from build123d import *

# Parameters (mm, degrees)
BOSS_EXTRUDE1_DEPTH = 3


with BuildPart() as part:
    # Base_Sketch → Boss-Extrude1 (new body)
    with BuildSketch(Plane.XY):
        with BuildLine():
            Line((-8.603981625, 52.439957176), (-8.603981625, 50.01533765))
            ThreePointArc((-8.603981625, 50.01533765), (-15.682612465, 48.266118202), (-22.437510505, 45.520551648))
            Line((-22.437510505, 45.520551648), (-23.862666105, 47.48211005))
            Line((-23.862666105, 47.48211005), (-24.825537526, 47.634613901))
            Line((-24.825537526, 47.634613901), (-37.631696962, 38.33039445))
            Line((-37.631696962, 38.33039445), (-37.784200813, 37.36752303))
            Line((-37.784200813, 37.36752303), (-36.359045213, 35.405964628))
            ThreePointArc((-36.359045213, 35.405964628), (-41.057612465, 29.830101554), (-44.908636245, 23.638462104))
            Line((-44.908636245, 23.638462104), (-47.214586445, 24.387710742))
            Line((-47.214586445, 24.387710742), (-48.083205302, 23.945127328))
            Line((-48.083205302, 23.945127328), (-52.974722942, 8.890584019))
            Line((-52.974722942, 8.890584019), (-52.532139528, 8.021965161))
            Line((-52.532139528, 8.021965161), (-50.226189328, 7.272716523))
            ThreePointArc((-50.226189328, 7.272716523), (-50.75, 0), (-50.226189328, -7.272716523))
            Line((-50.226189328, -7.272716523), (-52.532139528, -8.021965161))
            Line((-52.532139528, -8.021965161), (-52.974722942, -8.890584019))
            Line((-52.974722942, -8.890584019), (-48.083205302, -23.945127328))
            Line((-48.083205302, -23.945127328), (-47.214586445, -24.387710742))
            Line((-47.214586445, -24.387710742), (-44.908636245, -23.638462104))
            ThreePointArc((-44.908636245, -23.638462104), (-41.057612465, -29.830101554), (-36.359045213, -35.405964628))
            Line((-36.359045213, -35.405964628), (-37.784200813, -37.36752303))
            Line((-37.784200813, -37.36752303), (-37.631696962, -38.33039445))
            Line((-37.631696962, -38.33039445), (-24.825537526, -47.634613901))
            Line((-24.825537526, -47.634613901), (-23.862666105, -47.48211005))
            Line((-23.862666105, -47.48211005), (-22.437510505, -45.520551648))
            ThreePointArc((-22.437510505, -45.520551648), (-15.682612465, -48.266118202), (-8.603981625, -50.01533765))
            Line((-8.603981625, -50.01533765), (-8.603981625, -52.439957176))
            Line((-8.603981625, -52.439957176), (-7.914641797, -53.129297004))
            Line((-7.914641797, -53.129297004), (7.914641797, -53.129297004))
            Line((7.914641797, -53.129297004), (8.603981625, -52.439957176))
            Line((8.603981625, -52.439957176), (8.603981625, -50.01533765))
            ThreePointArc((8.603981625, -50.01533765), (15.682612465, -48.266118202), (22.437510505, -45.520551648))
            Line((22.437510505, -45.520551648), (23.862666105, -47.48211005))
            Line((23.862666105, -47.48211005), (24.825537526, -47.634613901))
            Line((24.825537526, -47.634613901), (37.631696962, -38.33039445))
            Line((37.631696962, -38.33039445), (37.784200813, -37.36752303))
            Line((37.784200813, -37.36752303), (36.359045213, -35.405964628))
            ThreePointArc((36.359045213, -35.405964628), (41.057612465, -29.830101554), (44.908636245, -23.638462104))
            Line((44.908636245, -23.638462104), (47.214586445, -24.387710742))
            Line((47.214586445, -24.387710742), (48.083205302, -23.945127328))
            Line((48.083205302, -23.945127328), (52.974722942, -8.890584019))
            Line((52.974722942, -8.890584019), (52.532139528, -8.021965161))
            Line((52.532139528, -8.021965161), (50.226189328, -7.272716523))
            ThreePointArc((50.226189328, -7.272716523), (50.75, 0), (50.226189328, 7.272716523))
            Line((50.226189328, 7.272716523), (52.532139528, 8.021965161))
            Line((52.532139528, 8.021965161), (52.974722942, 8.890584019))
            Line((52.974722942, 8.890584019), (48.083205302, 23.945127328))
            Line((48.083205302, 23.945127328), (47.214586445, 24.387710742))
            Line((47.214586445, 24.387710742), (44.908636245, 23.638462104))
            ThreePointArc((44.908636245, 23.638462104), (41.057612465, 29.830101554), (36.359045213, 35.405964628))
            Line((36.359045213, 35.405964628), (37.784200813, 37.36752303))
            Line((37.784200813, 37.36752303), (37.631696962, 38.33039445))
            Line((37.631696962, 38.33039445), (24.825537526, 47.634613901))
            Line((24.825537526, 47.634613901), (23.862666105, 47.48211005))
            Line((23.862666105, 47.48211005), (22.437510505, 45.520551648))
            ThreePointArc((22.437510505, 45.520551648), (15.682612465, 48.266118202), (8.603981625, 50.01533765))
            Line((8.603981625, 50.01533765), (8.603981625, 52.439957176))
            Line((8.603981625, 52.439957176), (7.914641797, 53.129297004))
            Line((7.914641797, 53.129297004), (-7.914641797, 53.129297004))
            Line((-7.914641797, 53.129297004), (-8.603981625, 52.439957176))
        make_face()
    extrude(amount=BOSS_EXTRUDE1_DEPTH)


solid = part.part
Verification items for the finished model (mm, model axes). A direction names the side the tool comes from. Coordinates: 2 decimals unless noted, no trailing zeros. Order: outer loops, then holes, each group sorted by start corner. A loop starts at its lowest first (then second) coordinate and runs counter-clockwise, first axis right, second up. Notation, with made-up numbers: M 15,-29 L 26,-29 A23 cw 26,10 Z; hole C 25.25,83.5 d4. An arc over 180 degrees is marked long. One line per item, written item: value. Start each with the question number.
Item 1: Gauge pin test, flat ends, axial feed: pin 1 (1.5 mm diameter, centred on y = -28.5, z = 2.5, fed in from -X); pin 2 (1 mm diameter, centred on x = 10.5, z = 2.5, fed in from -Y) (3 decimals); pin 3 (1.5 mm diameter, centred on x = -37.5, z = 1, fed in from -Y). Record the tip position at first contact, or that the pin passes through.
Item 2: Scan lines: probe 1 along X at (y, z) = (46, 2.6); probe 2 along X at (y, z) = (0.5, 1.4); probe 3 along Y at (x, z) = (44, 0.3). Record each from-to range of solid material in increasing order.
Item 3: Sectioned sample at A-A (y = -15). Enter the section's corners in (x, z), then the cut area to 3 significant figures.
Item 4: Mould release check, pull along Y, two halves, no side actions. Record for faces 6 (the flat face through (-8.604, -51, 1)), 7 (the flat face through (-51.395, 7.653, 1.479)), 8 (the flat face through (51.36, 7.64, 1.48)), 9 (the flat face through (-31.139, 43.048, 1.479)): released by +Y, released by -Y, zero draft, split by the parting line, or undercut.
Item 5: Access from +Z, -Z, +X, -X, +Y, -Y to the whole of each face (thin tool, end or side, straight path). Record for faces 1 (the flat face through (8.604, 51, 1)), 2 (the flat face through (-50.563, -16.312, 1.479)), 3 (the flat face through (-46.08, -24.02, 1.48)), 4 (the cylindrical face through (15.78, 48.234, 1.479)), 5 (the flat face through (8.604, -51, 1)).
Item 6: Sectioned sample at B-B (x = 42.5). Enter the section's corners in (y, z).
Conclusion:
1. pin 1: stops at x = -42.49
1. pin 2: stops at y = -49.755
1. pin 3: stops at y = -38.97
2. probe 1: x = -27.08 to -22.79, -21.44 to 21.44, 22.79 to 27.08
2. probe 2: x = -50.75 to 50.75
2. probe 3: y = -25.29 to 25.29
3. outline: M -50.99,0 L 50.99,0 L 50.99,3 L -50.99,3 Z
3. area: 306 mm^2
4. face 6: zero draft
4. face 7: undercut
4. face 8: undercut
4. face 9: released by +Y
5. face 1: +Z, -Z, +X, +Y
5. face 2: +Z, -Z, -X, -Y
5. face 3: +Z, -Z, -Y
5. face 4: +Z, -Z, +Y
5. face 5: +Z, -Z, +X, -Y
6. outline: M -27.74,0 L 27.74,0 L 27.74,3 L -27.74,3 Z
